Design review of the part built by this model. Coordinates are the model's own, in mm. Give positions to 0.01 mm unless a question says otherwise; leave off trailing zeros. Order: outer loops, then holes, each group sorted by start corner. A loop starts at its lowest first (then second) coordinate and runs counter-clockwise, first axis right, second up. Notation, with made-up numbers: M 42.25,-9.75 L 83.25,-9.75 A26 cw 83.25,19.25 Z; hole C 5.5,-15 d9. An arc over 180 degrees is marked long. Answer as a JSON object with one key per item and string values.
from build123d import *

# Parameters (mm, degrees)
SKETCH1_W                 = 19.05
SKETCH1_H                 = 103.886
BOSS_EXTRUDE1_DEPTH       = 6.35
M8_CLEARANCE_HOLE1_D      = 9
M8_CLEARANCE_HOLE1_DEPTH  = 21.082
M8_CLEARANCE_HOLE1_TIP    = 2.703872786
M10_CLEARANCE_HOLE1_D     = 11
M10_CLEARANCE_HOLE1_DEPTH = 21.082
M10_CLEARANCE_HOLE1_TIP   = 3.304733405


with BuildPart() as part:
    # Sketch1 → Boss-Extrude1 (new body)
    with BuildSketch(Plane.XY):
        with Locations((0, -84.724)):
            Rectangle(SKETCH1_W, SKETCH1_H)
    extrude(amount=BOSS_EXTRUDE1_DEPTH)

    # M8 Clearance Hole1
    with Locations(Plane.XY.offset(6.35)):
        with Locations((0, -127.142)):
            Hole(M8_CLEARANCE_HOLE1_D / 2, depth=M8_CLEARANCE_HOLE1_DEPTH)
            with Locations((0, 0, -(M8_CLEARANCE_HOLE1_DEPTH + M8_CLEARANCE_HOLE1_TIP / 2))):  # 118° drill point
                Cone(0, M8_CLEARANCE_HOLE1_D / 2, M8_CLEARANCE_HOLE1_TIP, mode=Mode.SUBTRACT)

    # M10 Clearance Hole1
    with Locations(Plane.XY.offset(6.35)):
        with Locations((0, -42.306)):
            Hole(M10_CLEARANCE_HOLE1_D / 2, depth=M10_CLEARANCE_HOLE1_DEPTH)
            with Locations((0, 0, -(M10_CLEARANCE_HOLE1_DEPTH + M10_CLEARANCE_HOLE1_TIP / 2))):  # 118° drill point
                Cone(0, M10_CLEARANCE_HOLE1_D / 2, M10_CLEARANCE_HOLE1_TIP, mode=Mode.SUBTRACT)


solid = part.part
(1) We need section B-B (y = -128.5). Write out the cut boundary in (x, z) (3 decimals).
Checked values:
{"outline": "M -9.525,0 L -4.29,0 L -4.29,6.35 L -9.525,6.35 Z; M 4.29,0 L 9.525,0 L 9.525,6.35 L 4.29,6.35 Z"}
(2) Draft analysis for pull direction Y (two halves, no side actions). For faces 1 (the flat face through (0, -136.667, 3)), 2 (the cylindrical face through (0.976, -131.535, 3.131)), 3 (the cylindrical face through (1.192, -47.675, 3.131)), 4 (the flat face through (-9.525, -85, 3)), state which applies: +Y half, -Y half, draft (parallel to the pull), parting line (faces both ways), or undercut.
Checked values:
{"face 1": "-Y half", "face 2": "undercut", "face 3": "undercut", "face 4": "draft"}
(3) We need section A-A (x = 0). Write out the cut boundary in (y, z).
Checked values:
{"outline": "M -136.67,0 L -131.64,0 L -131.64,6.35 L -136.67,6.35 Z; M -122.64,0 L -47.81,0 L -47.81,6.35 L -122.64,6.35 Z; M -36.81,0 L -32.78,0 L -32.78,6.35 L -36.81,6.35 Z"}
(4) To check wall thickness, follow L1, parallel to Y at x = 0, z = 3.5; L2, parallel to Y at x = 1.25, z = 5; L3, parallel to X at y = -44, z = 2.25 (3 decimals). State the ranges of each line that lie inside material, in increasing order. Write a range as from..to.
Checked values:
{"L1": "y = -136.67..-131.64, -122.64..-47.81, -36.81..-32.78", "L2": "y = -136.67..-131.46, -122.82..-47.66, -36.95..-32.78", "L3": "x = -9.525..-5.233, 5.233..9.525"}
(5) We need section C-C (z = 1). Write out the cut boundary in (x, y) (3 decimals).
Checked values:
{"outline": "M -9.525,-136.667 L 9.525,-136.667 L 9.525,-32.781 L -9.525,-32.781 Z; hole C 0,-42.306 d11; hole C 0,-127.142 d9"}
